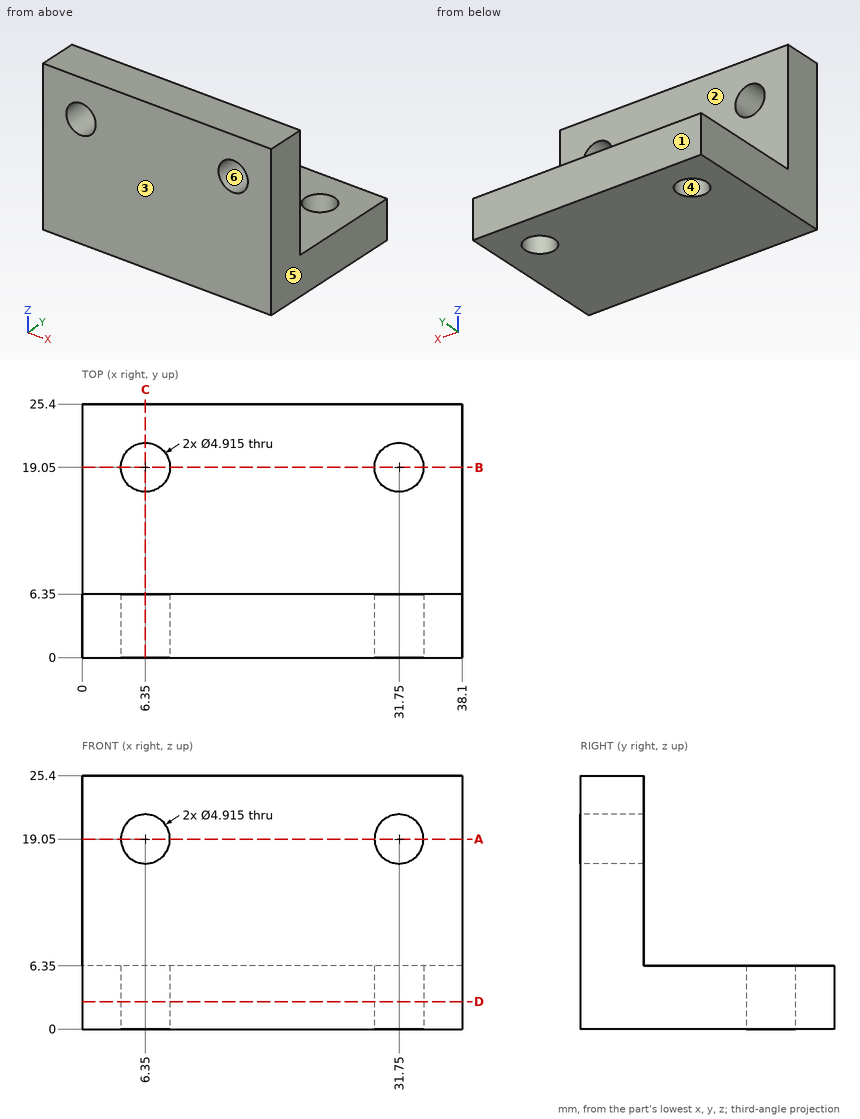
Job drawing, mm, ordinate dimensions from the low corner. One solid piece. A direction names the side the tool comes from. Give positions to 0.01 mm unless a question says otherwise; leave off trailing zeros. Loops run counter-clockwise (first coordinate to the right, second up) from the corner with the lowest first, then second, coordinate; pieces in that order, holes last. Notation, with made-up numbers: (-4.5, 58.5) -> (43.5, 58.5) arc R19 cw to (43.5, 95.5) -> close; hole circle Ø6 at (19, 73.25). An arc over 180 degrees is marked (long way). Use a Markdown table: item, result. Add a question column.
(1) Slice it at D-D on z = 2.75. Give the number of separate pieces and of enclosed holes in the cut face, and give its area (3 significant figures).
(2) Tool access for the marked faces 1 and 2: list every direction of +Z, -Z, +X, -X, +Y, -Y with a clear straight run to the whole face (end or side of a thin tool).
(3) Slice it at C-C on x = 6.35. List the corners of the cut face in (y, z), and give its area (3 significant figures).
(4) Slice it at A-A on z = 19.05. List the corners of the cut face in (x, y).
(5) Drop flat-ended pins along their axis: pin 1 Ø9.5 at (x, z) = (26, 12) entering from +Y; pin 2 Ø4 at (x, z) = (6.35, 19.05) entering from +Y. Give the stop position or say it passes through.
(6) Wall check: line 1 along X through (y, z) = (19, 5); line 2 along Y through (x, z) = (6.35, 4); line 3 along X through (y, z) = (5, 17) (1 decimal). Give the ranges that are in metal, low to high.
(7) Mould opens along X. For the marked faces 3, 4, 5 and 6 say: +X half, -X half, draft (parallel to the pull), parting line (faces both ways), or undercut.
Filled sheet:
| question | item | result |
|---|---|---|
| 1 | separate pieces | 1 |
| 1 | enclosed holes | 2 |
| 1 | area | 930 mm2 |
| 2 | face 1 | +Z, -Z, +X, -X, +Y |
| 2 | face 2 | +Z, +X, -X, +Y |
| 3 | outline | (0, 0) -> (16.59, 0) -> (16.59, 6.35) -> (6.35, 6.35) -> (6.35, 16.59) -> (0, 16.59) -> close; (0, 21.51) -> (6.35, 21.51) -> (6.35, 25.4) -> (0, 25.4) -> close; (21.51, 0) -> (25.4, 0) -> (25.4, 6.35) -> (21.51, 6.35) -> close |
| 3 | area | 220 mm2 |
| 4 | outline | (0, 0) -> (3.89, 0) -> (3.89, 6.35) -> (0, 6.35) -> close; (8.81, 0) -> (29.29, 0) -> (29.29, 6.35) -> (8.81, 6.35) -> close; (34.21, 0) -> (38.1, 0) -> (38.1, 6.35) -> (34.21, 6.35) -> close |
| 5 | pin 1 | y = 6.35 |
| 5 | pin 2 | through |
| 6 | line 1 | 0 to 3.89, 8.81 to 29.29, 34.21 to 38.1 |
| 6 | line 2 | 0 to 16.59, 21.51 to 25.4 |
| 6 | line 3 | 0 to 5, 7.7 to 30.4, 33.1 to 38.1 |
| 7 | face 3 | draft |
| 7 | face 4 | undercut |
| 7 | face 5 | +X half |
| 7 | face 6 | undercut |
